Input: part model. Units: mm. Frame: model coordinates. Give positions to 0.01 mm unless a question says otherwise; leave off trailing zeros. Loops run counter-clockwise (first coordinate to the right, second up) from the corner with the lowest first, then second, coordinate; pieces in that order, holes last. Notation, with made-up numbers: (79, -8) - (84, -8) arc R36 cw to (84, 26) - close; hole circle Ø10 at (29, 45). An arc over 180 degrees is marked (long way). Answer as a JSON object with one key per item and string values.
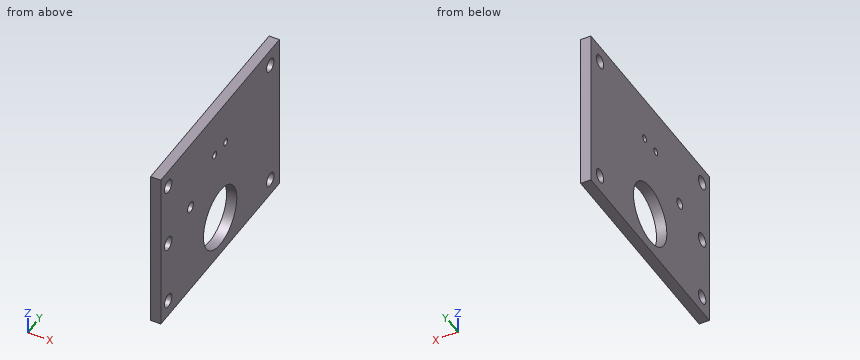
from build123d import *

# Parameters (mm, degrees)
SKETCH2_W            = 76.2
SKETCH2_H            = 101.6
BOSS_EXTRUDE1_DEPTH  = 4.7625
SKETCH3_R            = 3.175
CUT_EXTRUDE1_DEPTH   = 6.35
SKETCH3_4_R          = 3.175
SKETCH3_4_R_2        = 14.2875
SKETCH3_4_R_3        = 2.4892
CUT_EXTRUDE2_DEPTH   = 6.35
M6_CLEARANCE_HOLE1_D = 3.3


with BuildPart() as part:
    # Sketch2 → Boss-Extrude1 (new body)
    with BuildSketch(Plane(origin=(0, 0, 0), x_dir=(0, 0, -1), z_dir=(1, 0, 0))):
        Rectangle(SKETCH2_W, SKETCH2_H)
    extrude(amount=BOSS_EXTRUDE1_DEPTH)

    # Sketch3 → Cut-Extrude1 (cut)
    with BuildSketch(Plane(origin=(4.7625, 0, 0), x_dir=(0, 0, -1), z_dir=(1, 0, 0))):
        with Locations((30.2768, 42.9768)):
            Circle(SKETCH3_R)
    extrude(amount=-CUT_EXTRUDE1_DEPTH, mode=Mode.SUBTRACT)

    # Sketch3<4> → Cut-Extrude2 (cut)
    with BuildSketch(Plane(origin=(4.7625, 0, 0), x_dir=(0, 0, -1), z_dir=(1, 0, 0))):
        with Locations((30.2768, -44.5643)):
            Circle(SKETCH3_4_R)
        with Locations((30.2768, 42.9768)):
            Circle(SKETCH3_4_R)
        with Locations((-30.2768, 42.9768)):
            Circle(SKETCH3_4_R)
        with Locations((-30.2768, -44.5643)):
            Circle(SKETCH3_4_R)
        with Locations((18.9484, 0)):
            Circle(SKETCH3_4_R_2)
        with Locations((-5.1816, -25.4)):
            Circle(SKETCH3_4_R_3)
        with Locations((0, -44.5643)):
            Circle(SKETCH3_4_R)
    extrude(amount=-CUT_EXTRUDE2_DEPTH, mode=Mode.SUBTRACT)

    # M6 Clearance Hole1 (through all)
    with Locations(Plane(origin=(4.7625, 0, 0), x_dir=(0, 0, -1), z_dir=(1, 0, 0))):
        with Locations((-17.5641, 4.7625), (-17.5641, -4.7625)):
            Hole(M6_CLEARANCE_HOLE1_D / 2)


solid = part.part
Item 1: Cut plane B-B (y = -25.4). Return loops of the section in (x, z), then the cut area to 3 significant figures.
Geometry check:
{"outline": "(0, -38.1) - (4.76, -38.1) - (4.76, 2.69) - (0, 2.69) - close; (0, 7.67) - (4.76, 7.67) - (4.76, 38.1) - (0, 38.1) - close", "area": "339 mm2"}
Item 2: Cut plane C-C (x = 2.1). Give the number of separate pieces and of enclosed holes in the cut face, then the cut area to 3 significant figures.
Geometry check:
{"separate pieces": "1", "enclosed holes": "9", "area": "6,910 mm2"}
Item 3: Material intervals for line 1 (Y direction, x = 3.65, z = 0); line 2 (Y direction, x = 2.65, z = -27.5); line 3 (Y direction, x = 0.5, z = -26), sorted ascending. Write a range as [from, to].
Geometry check:
{"line 1": "y = [-50.8, -47.74], [-41.39, 50.8]", "line 2": "y = [-50.8, -46.1], [-43.02, -11.45], [11.45, 41.44], [44.52, 50.8]", "line 3": "y = [-50.8, -12.43], [12.43, 50.8]"}
Item 4: Cut plane A-A (z = 0). Return loops of the section in (x, y).
Geometry check:
{"outline": "(0, -50.8) - (4.76, -50.8) - (4.76, -47.74) - (0, -47.74) - close; (0, -41.39) - (4.76, -41.39) - (4.76, 50.8) - (0, 50.8) - close"}
Item 5: Contact query for a flat-ended pin moving along its axis: P1, Ø5, axis at y = -44.56, z = 30.28, coming from the -X side. Output: stop coordinate, or through.
Geometry check:
{"P1": "passes through"}
